from build123d import *

# Parameters (mm, degrees)
BOSS_EXTRUDE1_DEPTH = 3
SKETCH2_W           = 21
SKETCH2_H           = 3
CUT_EXTRUDE1_DEPTH  = 3


with BuildPart() as part:
    # Sketch1 → Boss-Extrude1 (new body)
    with BuildSketch(Plane(origin=(0, 0, 0), x_dir=(1, 0, 0), z_dir=(0, 1, 0))):
        Polygon((-35, -35), (-17.5, -35), (-17.5, -38), (17.5, -38), (17.5, -35), (35, -35), (35, -17.5), (38, -17.5), (38, 17.5), (35, 17.5), (35, 35), (17.5, 35), (17.5, 38), (-17.5, 38), (-17.5, 35), (-35, 35), (-35, 17.5), (-38, 17.5), (-38, -17.5), (-35, -17.5), align=None)
    extrude(amount=BOSS_EXTRUDE1_DEPTH)

    # Sketch2 → Cut-Extrude1 (cut)
    with BuildSketch(Plane(origin=(0, 3, 0), x_dir=(1, 0, 0), z_dir=(0, 1, 0))):
        Rectangle(SKETCH2_W, SKETCH2_H)
    extrude(amount=-CUT_EXTRUDE1_DEPTH, mode=Mode.SUBTRACT)


solid = part.part
Verification items for the finished model (mm, model axes). A direction names the side the tool comes from. Coordinates: 2 decimals unless noted, no trailing zeros. Loops run counter-clockwise (first coordinate to the right, second up) from the corner with the lowest first, then second, coordinate; pieces in that order, holes last. Notation, with made-up numbers: M 72.25,9.25 L 113.25,9.25 A24 cw 113.25,35.25 Z; hole C -1,65 d6. An arc over 180 degrees is marked long. One line per item, written item: value.
1. Section check A-A on x = -3. Record the cut outline in (y, z).
Answers follow:
outline: M 0,-38 L 3,-38 L 3,-1.5 L 0,-1.5 Z; M 0,1.5 L 3,1.5 L 3,38 L 0,38 Z
2. Set-up check for faces 4 (the flat face through (37, 1, -17.5)), 5 (the flat face through (-17.5, 1, -37)), 6 (the flat face through (17.5, 1, 37)): record each of +Z, -Z, +X, -X, +Y, -Y from which the full face is reachable in a straight line by a thin tool's end or side.
Answers follow:
face 4: -Z, +X, +Y, -Y
face 5: -Z, -X, +Y, -Y
face 6: +Z, +X, +Y, -Y
3. Section check D-D on x = -29. Record the cut outline in (y, z).
Answers follow:
outline: M 0,-35 L 3,-35 L 3,35 L 0,35 Z
4. Section check B-B on y = 0.5. Record the cut outline in (x, z), plus the area to 3 significant figures.
Answers follow:
outline: M -38,-17.5 L -35,-17.5 L -35,-35 L -17.5,-35 L -17.5,-38 L 17.5,-38 L 17.5,-35 L 35,-35 L 35,-17.5 L 38,-17.5 L 38,17.5 L 35,17.5 L 35,35 L 17.5,35 L 17.5,38 L -17.5,38 L -17.5,35 L -35,35 L -35,17.5 L -38,17.5 Z; hole M -10.5,-1.5 L 10.5,-1.5 L 10.5,1.5 L -10.5,1.5 Z
area: 5,260 mm^2
5. Material ranges on line 1 along Z through (x, y) = (9, 2); line 2 along Z through (x, y) = (33, 1.9), recorded low to high. Write a range as from..to.
Answers follow:
line 1: -38..-1.5, 1.5..38
line 2: -35..35
6. Section check C-C on z = 22.5. Record the cut outline in (x, y).
Answers follow:
outline: M -35,0 L 35,0 L 35,3 L -35,3 Z
7. Mould release check, pull along X, two halves, no side actions. Record for faces 1 (the flat face through (0, 2, 1.5)), 2 (the flat face through (0, 1, 38)), 3 (the flat face through (35, 1, -26)): pulls with the +X half, pulls with the -X half, needs draft (parallel to the pull), parting line crosses it, or undercut.
Answers follow:
face 1: undercut
face 2: needs draft
face 3: pulls with the +X half
8. Gauge pin test, flat ends, axial feed: P1, Ø3, axis at x = -19.5, z = 6.5, coming from the -Y side; P2, Ø1.5, axis at x = 30.5, y = 1, coming from the -Z side; P3, Ø0.9, axis at y = 1.5, z = -30.5, coming from the -X side; P4, Ø1.5, axis at x = 37, y = 1, coming from the +Z side. Record the tip position at first contact, or that the pin passes through.
Answers follow:
P1: y = 0
P2: z = -35
P3: x = -35
P4: z = 17.5
